from build123d import *

# Parameters (mm, degrees)
F1_DEPTH = 2.5
F2_SIZE  = 2.49999
F4_DEPTH = 2.5


# Not quite as in the source:
# - a fillet or chamfer is up to 0.001 mm smaller than in the source, because OpenCascade refuses the exact size


with BuildPart() as f1:
    # F0 (on Top) → F1 (new body, symmetric)
    with BuildSketch(Plane.XY):
        Polygon((-3.1822135206, 54.0976710618), (-3.1822135206, -76.2216448784), (3.7883522455, -76.2216448784), (3.7883522455, 54.0976710618), (0, 62.2805096209), align=None)
    extrude(amount=F1_DEPTH, both=True)

    # F2 (size 2.5 in the source; OpenCascade refuses exactly that, so slightly less here)
    f2_edges = [f1.edges().sort_by_distance(p)[0] for p in [
        (-1.591107, 58.18909, -2.5),
        (-3.182214, -11.061987, -2.5),
        (0.303069, -76.221645, -2.5),
        (3.788352, -11.061987, -2.5),
        (1.894176, 58.18909, -2.5),
        (-1.591107, 58.18909, 2.5),
        (-3.182214, -11.061987, 2.5),
        (0.303069, -76.221645, 2.5),
        (3.788352, -11.061987, 2.5),
        (1.894176, 58.18909, 2.5),
    ]]
    chamfer(f2_edges, length=F2_SIZE)

    # F3 (on Top) → F4 (join, symmetric)
    with BuildSketch(Plane.XY):
        with BuildLine():
            Line((-7.067034021, -69.0257325768), (-7.067034021, -76.5438452363))
            Line((-7.067034021, -76.5438452363), (7.9692080617, -76.5438452363))
            Line((7.9692080617, -76.5438452363), (7.9692080617, -69.0257325768))
            ThreePointArc((7.9692080617, -69.0257325768), (2.0355302464, -56.380771616), (0, -42.5619371235))
            ThreePointArc((0, -42.5619371235), (-1.7971813817, -56.2575152388), (-7.067034021, -69.0257325768))
        make_face()
    extrude(amount=F4_DEPTH, both=True)


solid = f1.part
Design review of the part built by this model. Coordinates are the model's own, in mm. A direction names the side the tool comes from. Round coordinates to 2 decimals unless told otherwise and drop trailing zeros. Write each loop counter-clockwise with the first axis right and the second up, starting at its lowest first coordinate (ties: lowest second). Pieces come first, ordered by that corner, then holes.
Item 1: Wall thickness on L1, parallel to Y at x = 1.75, z = -1.85; L2, parallel to X at y = -33, z = -0.85; L3, parallel to X at y = 29.5, z = 0.6: over which ranges is each line inside the solid? List them lowest first.
Item 2: Consider section B-B on z = -1.4. Give the boundary of the cut face in (x, y).
Item 3: For faces 1 (the flat face through (-1.91, -2.48, 1.27)), 2 (the flat face through (2.52, -4.38, -1.27)), 3 (the flat face through (2.52, -4.38, 1.27)), list the 3-axis set-ups (+Z, -Z, +X, -X, +Y, -Y) from which the entire face can be reached by the end or side of a thin tool; tool diameter is ignored.
Item 4: Consider section C-C on x = 5.5. Give the boundary of the cut face in (y, z), and give its area (3 significant figures).
Check values:
1. L1: y = -76.54 to 54.1
1. L2: x = -2.33 to 2.94
1. L3: x = -2.58 to 3.19
2. outline: (-7.07, -76.54) - (7.97, -76.54) - (7.97, -69.03) arc R47.92 cw to (2.39, -57.5) - (2.39, 53.79) - (0.11, 58.71) - (-1.78, 53.84) - (-1.78, -56.2) arc R53.08 cw to (-7.07, -69.03) - close
3. face 1: +Z, -X, +Y
3. face 2: -Z, +X, +Y
3. face 3: +Z, +X, +Y
4. outline: (-76.54, -2.5) - (-64.85, -2.5) - (-64.85, 2.5) - (-76.54, 2.5) - close
4. area: 58.5 mm2
